Work out the finished part from the listing and answer in its coordinate system (mm). Face numbers are marked on the shaded views. Round coordinates to 2 decimals unless told otherwise and drop trailing zeros. Order: outer loops, then holes, each group sorted by start corner. A loop starts at its lowest first (then second) coordinate and runs counter-clockwise, first axis right, second up. Notation, with made-up numbers: (-15.5, 17.5) - (13.5, 17.5) arc R18 cw to (13.5, 23.5) - close; hole circle Ø6 at (56, 50). An arc over 180 degrees is marked (long way). One line per question, with ' | ' between items. Start each with the question number.
Autodesk Inventor part; units mm, degrees
ref_plane "YZ Plane" through (0, 0, 0) normal (1, 0, 0) x (0, 1, 0)
ref_plane "XZ Plane" through (0, 0, 0) normal (0, 1, 0) x (-1, 0, 0)
ref_plane "XY Plane" through (0, 0, 0) normal (0, 0, 1) x (1, 0, 0)
ref_plane "Arbeitsebene1" through (-0.0002, 0, 0) normal (0, 0, 1) x (1, 0, 0)
sketch "Skizze1" plane through (-0.0002, 0, 0) normal (0, 0, 1) x (1, 0, 0)
  circle A0 centre (13.85, 6.86) radius 1.5
  circle A1 centre (0.85, 31.86) radius 1.5
  circle A2 centre (13.85, 31.86) radius 1.5
  circle A3 centre (0.85, 6.86) radius 1.5
  circle A4 centre (5.0933, 19.36) radius 5.5
  line L0 (-3.07, 5.49) -> (-3.07, 33.23)
  line L1 (-3.07, 5.49) -> (-16.87, 5.49)
  line L2 (-16.87, 13.31) -> (-16.87, 5.49)
  line L3 (-16.8476, 13.31) -> (-16.87, 13.31)
  line L4 (-16.8476, 25.41) -> (-16.8476, 13.31)
  line L5 (-16.87, 25.41) -> (-16.8476, 25.41)
  line L6 (-16.87, 33.23) -> (-16.87, 25.41)
  line L7 (-3.07, 33.23) -> (-16.87, 33.23)
  line L8 (-16.87, 40.13) -> (-16.87, 44.21)
  line L9 (-20.77, 36.23) -> (-16.87, 40.13)
  line L10 (-24.85, 36.23) -> (-20.77, 36.23)
  line L11 (-24.85, 2.49) -> (-24.85, 36.23)
  line L12 (-20.77, 2.49) -> (-24.85, 2.49)
  line L13 (-16.87, -1.41) -> (-20.77, 2.49)
  line L14 (-16.87, -1.41) -> (-16.87, -5.49)
  line L15 (-16.87, -5.49) -> (16.87, -5.49)
  line L16 (16.87, -5.49) -> (16.87, -1.41)
  line L17 (20.77, 2.49) -> (16.87, -1.41)
  line L18 (24.85, 2.49) -> (20.77, 2.49)
  line L19 (24.85, 36.23) -> (24.85, 2.49)
  line L20 (20.77, 36.23) -> (24.85, 36.23)
  line L21 (16.87, 40.13) -> (20.77, 36.23)
  line L22 (16.87, 44.21) -> (16.87, 40.13)
  line L23 (-16.87, 44.21) -> (16.87, 44.21)
  line L24 (16.97, 36.33) -> (16.97, 2.39)
  line L25 (-16.97, 36.33) -> (16.97, 36.33) construction
  line L26 (-16.97, 2.39) -> (-16.97, 36.33)
  line L27 (16.97, 2.39) -> (-16.97, 2.39) construction
  line L28 (16.97, 2.39) -> (-16.97, 2.39)
  line L29 (16.47, 35.83) -> (16.47, 2.89)
  line L30 (16.47, 2.89) -> (-16.47, 2.89)
  line L31 (-16.47, 2.89) -> (-16.47, 35.83)
  line L32 (-16.47, 35.83) -> (16.47, 35.83)
  line L33 (-2.57, 35.83) -> (-2.57, 2.89)
  circle A5 centre (5.0933, 19.36) radius 3.505
  circle A6 centre (5.0933, 19.36) radius 3
  point P0 (0.0002, 0)
  point P1 (16.47, 19.36)
extrude "Extrusion1" add sketch "Skizze1" along normal blind 5 contours A4 | L33 L32 L29 L30 | A5
sketch "Skizze5" plane through (16.4698, 2.89, 0) normal (1, 0, 0) x (0, 0, -1)
  line L0 (-23, 19.975) -> (-4.8046, 19.975)
  line L1 (-23, 12.965) -> (-4.8046, 12.965)
  circle A0 centre (-2.5, 20.475) radius 1.4
  circle A1 centre (-2.5, 12.465) radius 1.4
  line L2 (-2.5, 20.475) -> (-2.5, 12.465) construction
  line L3 (0, 32.94) -> (-5, 32.94)
  line L4 (-5, 0) -> (-5, 32.94)
  line L5 (-5, 16.47) -> (0, 16.47) construction
  line L6 (0, 0) -> (0, 32.94)
  point P0 (0, -2.89)
  point P1 (-2.5, 32.94)
  point P2 (-2.5, 16.47)
  dimension "d19" = 2.8
  dimension "d20" = 2.8
  dimension "d21" = 0.5
  dimension "d22" = 0.5
extrude "Extrusion4" cut sketch "Skizze5" against normal through all
equation "\"d22\" = d21"
properties part number "30_Cube_Z_Focus_NEMA8_captive_micrometerscrewbase_v0"
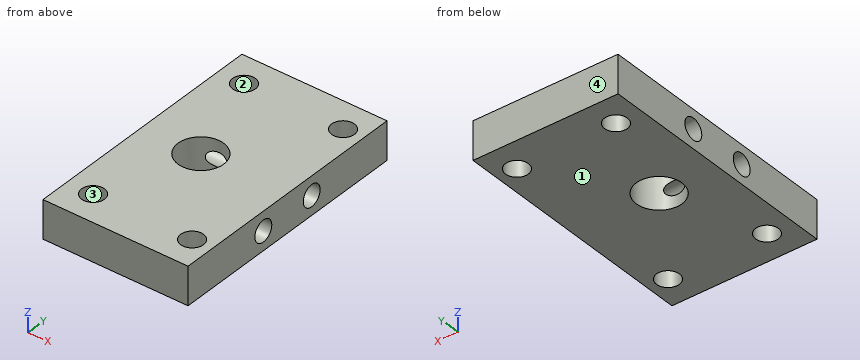
1) Straight lines are drawn through the part: line 1 (Y direction, x = 11.25, z = 2.5) (3 decimals); line 2 (Y direction, x = 2, z = 4.65); line 3 (X direction, y = 6.5, z = 1.9). For each, find the intervals that lie inside material, in ascending order.
2) Section D-D on y = 21.5 is taken. Give the vertices of the cut face in (x, z).
3) Section B-B on y = 6.86 is taken. Give the vertices of the cut face in (x, z), and give its area (3 significant figures).
4) Section C-C on x = 5.5 is taken. Give the vertices of the cut face in (y, z) (3 decimals), and give its area (3 significant figures).
5) Section A-A on z = 3.15 is taken. Give the vertices of the cut face in (x, y), and give its area (3 significant figures).
6) Determine the mould class of the marked faces 1, 2, 3 and 4 for opening direction Y: released by +Y, released by -Y, zero draft, split by the parting line, or undercut.
Recorded:
1) line 1: y = 2.89 to 13.955, 16.755 to 21.965, 24.765 to 35.83 | line 2: y = 2.89 to 5.9, 7.82 to 30.9, 32.82 to 35.83 | line 3: x = -2.57 to -0.61, 2.31 to 12.39, 15.31 to 16.47
2) outline: (-2.57, 0) - (2.99, 0) - (2.99, 5) - (-2.57, 5) - close; (7.2, 0) - (16.47, 0) - (16.47, 5) - (7.2, 5) - close
3) outline: (-2.57, 0) - (-0.65, 0) - (-0.65, 5) - (-2.57, 5) - close; (2.35, 0) - (12.35, 0) - (12.35, 5) - (2.35, 5) - close; (15.35, 0) - (16.47, 0) - (16.47, 5) - (15.35, 5) - close | area: 65.2 mm²
4) outline: (2.89, 0) - (16.388, 0) - (16.388, 1.555) arc R1.4 cw (long way) to (16.388, 3.445) - (16.388, 5) - (2.89, 5) - close; (22.332, 0) - (35.83, 0) - (35.83, 5) - (22.332, 5) - (22.332, 3.445) arc R1.4 cw (long way) to (22.332, 1.555) - close | area: 124 mm²
5) outline: (-2.57, 2.89) - (16.47, 2.89) - (16.47, 14.12) - (-2.57, 14.12) - close; (-2.57, 16.59) - (3.93, 16.59) arc R3 cw to (3.93, 22.13) - (-2.57, 22.13) - close; (-2.57, 24.6) - (16.47, 24.6) - (16.47, 35.83) - (-2.57, 35.83) - close; (6.26, 16.59) - (16.47, 16.59) - (16.47, 22.13) - (6.26, 22.13) arc R3 cw to start; hole circle Ø3 at (0.85, 6.86); hole circle Ø3 at (0.85, 31.86); hole circle Ø3 at (13.85, 6.86); hole circle Ø3 at (13.85, 31.86) | area: 477 mm²
6) face 1: zero draft | face 2: undercut | face 3: undercut | face 4: released by +Y
